Could you check a few things on this drawing? It's one solid part, dimensions in mm from its lowest x, y, z. A direction names the side the tool comes from. Coordinates: 2 decimals unless noted, no trailing zeros. Order: outer loops, then holes, each group sorted by start corner. A loop starts at its lowest first (then second) coordinate and runs counter-clockwise, first axis right, second up.
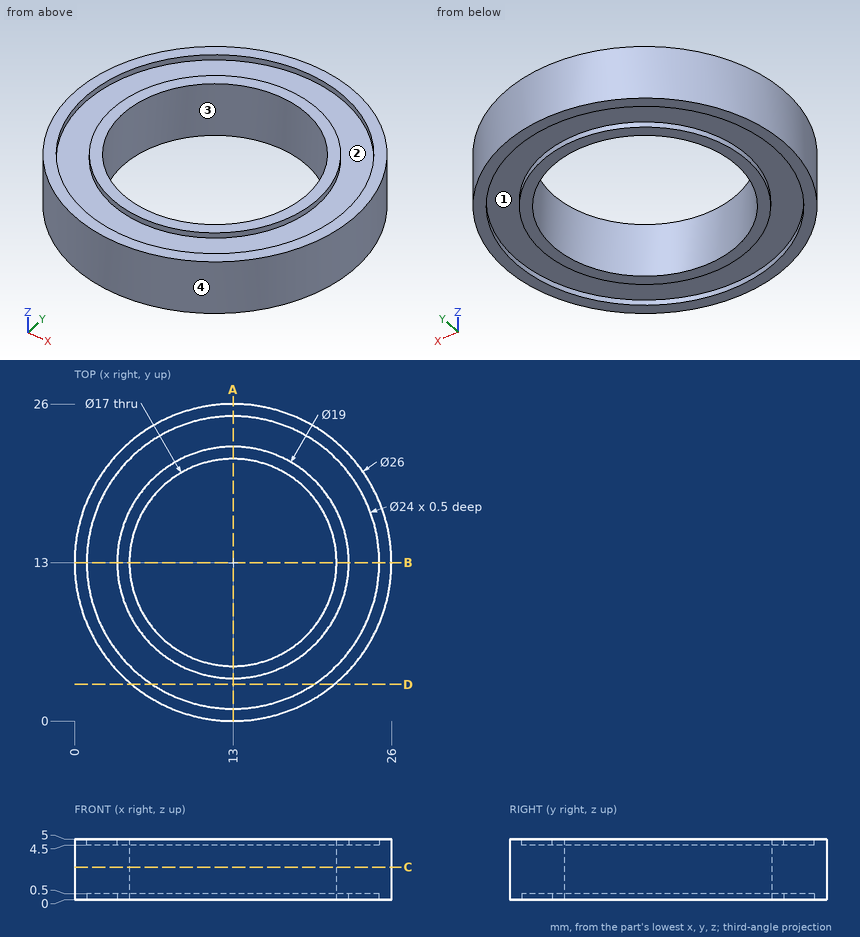
Item 1: For pin 1 Ø1 at (x, z) = (22, 2.5) entering from +Y; pin 2 Ø3 at (x, z) = (19.5, 0.5) entering from -Y; pin 3 Ø3 at (x, z) = (17, 1) entering from -Y; pin 4 Ø7 at (x, y) = (13, 7.5) entering from +Z, each with a flat end and sliding along its axis, tell me the tip position at first contact or that it passes through.
Item 2: Which directions (+Z, -Z, +X, -X, +Y, -Y) give clear straight access to the entire face, cutting with the end or side of a thin tool? Please do the marked faces 1 and 2.
Item 3: Suppose I cut it at A-A (x = 13). List the corners of the cut face in (y, z) for me, and give its area (3 significant figures).
Item 4: I need wall thicknesses on line 1 (Y direction, x = 13, z = 4.8); line 2 (Y direction, x = 13, z = 1.5); line 3 (Z direction, x = 24.5, y = 12.25). Which ranges of each line are inside material? Lowest first, please.
Item 5: Suppose I cut it at D-D (y = 3). List the corners of the cut face in (x, z) for me.
Item 6: Suppose I cut it at C-C (z = 2.7). List the corners of the cut face in (x, y) for me, and give its area (3 significant figures).
Item 7: Thinking about a two-plate mould opening in Y: for the marked faces 3 and 4, which applies, +Y half, -Y half, draft (parallel to the pull), parting line (faces both ways), or undercut?
Geometry results:
1. pin 1: stops at y = 22.84
1. pin 2: stops at y = 1
1. pin 3: stops at y = 0.24
1. pin 4: stops at z = 5
2. face 1: -Z
2. face 2: +Z
3. outline: (0, 0) - (1, 0) - (1, 0.5) - (3.5, 0.5) - (3.5, 0) - (4.5, 0) - (4.5, 5) - (3.5, 5) - (3.5, 4.5) - (1, 4.5) - (1, 5) - (0, 5) - close; (21.5, 0) - (22.5, 0) - (22.5, 0.5) - (25, 0.5) - (25, 0) - (26, 0) - (26, 5) - (25, 5) - (25, 4.5) - (22.5, 4.5) - (22.5, 5) - (21.5, 5) - close
3. area: 40.0 mm2
4. line 1: y = 0 to 1, 3.5 to 4.5, 21.5 to 22.5, 25 to 26
4. line 2: y = 0 to 4.5, 21.5 to 26
4. line 3: z = 0.5 to 4.5
5. outline: (4.69, 0) - (6.37, 0) - (6.37, 0.5) - (19.63, 0.5) - (19.63, 0) - (21.31, 0) - (21.31, 5) - (19.63, 5) - (19.63, 4.5) - (6.37, 4.5) - (6.37, 5) - (4.69, 5) - close
6. outline: circle Ø26 at (13, 13); hole circle Ø17 at (13, 13)
6. area: 304 mm2
7. face 3: undercut
7. face 4: parting line
